Could you check a few things on this model? Use its own coordinates, in mm. Face numbers are marked on the shaded views. A direction names the side the tool comes from. Give positions to 0.01 mm unless a question says otherwise; leave off trailing zeros. Order: outer loops, then holes, each group sorted by start corner. A loop starts at its lowest first (then second) coordinate and runs counter-clockwise, first axis right, second up. Notation, with made-up numbers: (87.5, 46) -> (141.5, 46) arc R13 cw to (141.5, 51) -> close; hole circle Ø10 at (55.25, 36). An arc over 180 degrees is marked (long way). Use one line per item in the form item = value. Start each with the question number.
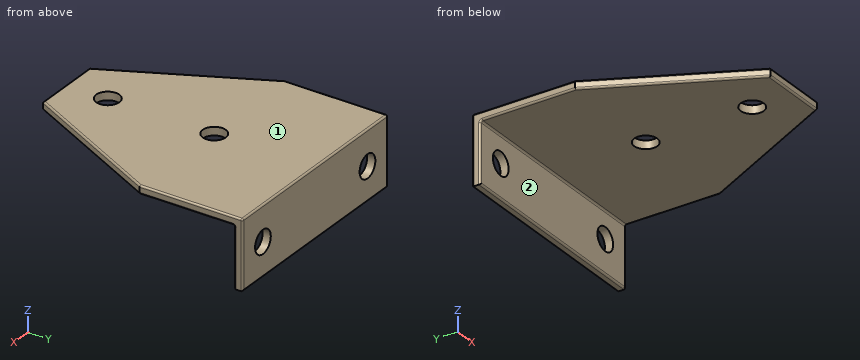
from build123d import *

# Parameters (mm, degrees)
SALIENTE_EXTRUIR1_DEPTH       = 4.8
CROQUIS2_W                    = 125
CROQUIS2_H                    = 4.8
SALIENTE_EXTRUIR2_DEPTH       = 35.2
REDONDEO1_R                   = 1
TALADRO_DE_MARGEN_PARA_M121_D = 13.5
TALADRO_DE_MARGEN_PARA_M122_D = 13.5


with BuildPart() as part:
    # Croquis1 → Saliente-Extruir1 (new body)
    with BuildSketch(Plane.XY):
        Polygon((-912.5, -63.6), (-912.5, -123.6), (-870, -208.6), (-830, -208.6), (-787.5, -123.6), (-787.5, -63.6), align=None)
    extrude(amount=-SALIENTE_EXTRUIR1_DEPTH)

    # Croquis2 → Saliente-Extruir2 (add)
    with BuildSketch(Plane(origin=(0, 0, -4.8), x_dir=(-1, 0, 0), z_dir=(0, 0, -1))):
        with Locations((850, -66)):
            Rectangle(CROQUIS2_W, CROQUIS2_H)
    extrude(amount=SALIENTE_EXTRUIR2_DEPTH)

    # Redondeo1
    redondeo1_edges = [part.edges().sort_by_distance(p)[0] for p in [
        (-912.5, -63.6, -20),
        (-787.5, -63.6, -20),
        (-912.5, -96, -4.8),
        (-891.25, -166.1, -4.8),
        (-850, -68.4, -4.8),
        (-787.5, -68.4, -22.4),
        (-912.5, -68.4, -22.4),
        (-850, -68.4, -40),
        (-850, -63.6, -40),
        (-850, -208.6, -4.8),
        (-808.75, -166.1, -4.8),
        (-850, -208.6, 0),
        (-891.25, -166.1, 0),
        (-912.5, -93.6, 0),
        (-850, -63.6, 0),
        (-787.5, -93.6, 0),
        (-808.75, -166.1, 0),
        (-787.5, -96, -4.8),
    ]]
    fillet(redondeo1_edges, radius=REDONDEO1_R)

    # Taladro de margen para M121 (through all)
    with Locations(Plane(origin=(0, -63.6, 0), x_dir=(1, 0, 0), z_dir=(0, 1, 0))):
        with Locations((-895, 20.5), (-805, 20.5)):
            Hole(TALADRO_DE_MARGEN_PARA_M121_D / 2)

    # Taladro de margen para M122 (through all)
    with Locations(Plane.XY):
        with Locations((-850, -122.4), (-850, -184.4)):
            Hole(TALADRO_DE_MARGEN_PARA_M122_D / 2)


solid = part.part
(1) Which directions (+Z, -Z, +X, -X, +Y, -Y) give clear straight access to the entire face, cutting with the end or side of a thin tool? Please do the marked faces 1 and 2.
(2) I'm going to push flat-ended pins straight in: pin 1 Ø17.5 at (x, z) = (-895, -20.5) entering from -Y; pin 2 Ø8 at (x, y) = (-880.5, -105) entering from -Z. Where does each tip first touch, or does it pass through?
(3) Imagine slicing it at B-B (x = -850). Write out the boundary of the cut face in (y, z).
(4) Imagine slicing it at C-C (z = -29.5). Write out the boundary of the cut face in (x, y), plus the area to 3 significant figures.
(5) Imagine slicing it at A-A (z = -20.5). Write out the boundary of the cut face in (x, y), plus the area to 3 significant figures.
(6) Please list where these lines run through material, in increasing order: probe 1 along Y at (x, z) = (-850, -2); probe 2 along X at (y, z) = (-67, -20.5); probe 3 along Z at (x, y) = (-805, -65.25).
Calculated:
q1.face_1 = +Z, +X, -X, +Y, -Y
q1.face_2 = -Z, +X, -X, -Y
q2.pin_1 = -68.4
q2.pin_2 = -4.8
q3.outline = (-208.6, -3.8) arc R1 ccw to (-207.6, -4.8) -> (-191.15, -4.8) -> (-191.15, 0) -> (-207.6, 0) arc R1 ccw to (-208.6, -1) -> close; (-177.65, -4.8) -> (-129.15, -4.8) -> (-129.15, 0) -> (-177.65, 0) -> close; (-115.65, -4.8) -> (-69.4, -4.8) arc R1 cw to (-68.4, -5.8) -> (-68.4, -39) arc R1 ccw to (-67.4, -40) -> (-64.6, -40) arc R1 ccw to (-63.6, -39) -> (-63.6, -1) arc R1 ccw to (-64.6, 0) -> (-115.65, 0) -> close
q4.outline = (-912.5, -67.4) arc R1 ccw to (-911.5, -68.4) -> (-788.5, -68.4) arc R1 ccw to (-787.5, -67.4) -> (-787.5, -64.6) arc R1 ccw to (-788.5, -63.6) -> (-911.5, -63.6) arc R1 ccw to (-912.5, -64.6) -> close
q4.area = 599 mm2
q5.outline = (-912.5, -67.4) arc R1 ccw to (-911.5, -68.4) -> (-901.75, -68.4) -> (-901.75, -63.6) -> (-911.5, -63.6) arc R1 ccw to (-912.5, -64.6) -> close; (-888.25, -68.4) -> (-811.75, -68.4) -> (-811.75, -63.6) -> (-888.25, -63.6) -> close; (-798.25, -68.4) -> (-788.5, -68.4) arc R1 ccw to (-787.5, -67.4) -> (-787.5, -64.6) arc R1 ccw to (-788.5, -63.6) -> (-798.25, -63.6) -> close
q5.area = 470 mm2
q6.probe_1 = -208.6 to -191.15, -177.65 to -129.15, -115.65 to -63.6
q6.probe_2 = -912.5 to -901.75, -888.25 to -811.75, -798.25 to -787.5
q6.probe_3 = -40 to -27.25, -13.75 to 0
